```python
from build123d import *

# Parameters (mm, degrees)
SKETCH1_R             = 3.9
SKETCH1_R_2           = 1.5
BOSS_EXTRUDE1_DEPTH   = 10.061552014
BOSS_EXTRUDE1_2_DEPTH = 10.061552014
BOSS_EXTRUDE1_3_DEPTH = 10.061552014
BOSS_EXTRUDE1_4_DEPTH = 10.061552014
BOSS_EXTRUDE2_START   = 1.861552
SKETCH2_R             = 3.9
SKETCH2_R_2           = 9.3
BOSS_EXTRUDE2_DEPTH   = 10
CUT_EXTRUDE1_DEPTH    = 25
CUT_EXTRUDE2_DEPTH    = 72.170463178
SKETCH5_W             = 10
SKETCH5_H             = 10
SKETCH5_R             = 2
BOSS_EXTRUDE3_DEPTH   = 10


with BuildPart() as part:
    # Sketch1 → Boss-Extrude1 (new body)
    with BuildSketch(Plane.XY):
        with Locations(Location((-49, 7.83595021, 0), (0, 0, 180))):
            Circle(SKETCH1_R)
        with Locations(Location((-49, 7.83595021, 0), (0, 0, 180))):
            Circle(SKETCH1_R_2, mode=Mode.SUBTRACT)
    extrude(amount=BOSS_EXTRUDE1_DEPTH)



with BuildPart() as body_2:
    # Sketch1 → Boss-Extrude1 2 (new body)
    with BuildSketch(Plane.XY):
        with Locations(Location((-49, 35.83595021, 0), (0, 0, 180))):
            Circle(SKETCH1_R)
        with Locations(Location((-49, 35.83595021, 0), (0, 0, 180))):
            Circle(SKETCH1_R_2, mode=Mode.SUBTRACT)
    extrude(amount=BOSS_EXTRUDE1_2_DEPTH)


with BuildPart() as body_3:
    # Sketch1 → Boss-Extrude1 3 (new body)
    with BuildSketch(Plane.XY):
        with Locations(Location((-9, 35.83595021, 0), (0, 0, 180))):
            Circle(SKETCH1_R)
        with Locations(Location((-9, 35.83595021, 0), (0, 0, 180))):
            Circle(SKETCH1_R_2, mode=Mode.SUBTRACT)
    extrude(amount=BOSS_EXTRUDE1_3_DEPTH)


with BuildPart() as body_4:
    # Sketch1 → Boss-Extrude1 4 (new body)
    with BuildSketch(Plane.XY):
        with Locations(Location((-9, 7.83595021, 0), (0, 0, 180))):
            Circle(SKETCH1_R)
        with Locations(Location((-9, 7.83595021, 0), (0, 0, 180))):
            Circle(SKETCH1_R_2, mode=Mode.SUBTRACT)
    extrude(amount=BOSS_EXTRUDE1_4_DEPTH)


with BuildPart() as part_1:
    add(part.part)

    add(body_2.part)  # Boss-Extrude2 merges body 2

    add(body_3.part)  # Boss-Extrude2 merges body 3

    add(body_4.part)  # Boss-Extrude2 merges body 4
    # Sketch2 → Boss-Extrude2 (add)
    with BuildSketch(Plane.XY.offset(-1.8).offset(BOSS_EXTRUDE2_START)):
        Polygon((-58, 1.83595021), (0, 1.83595021), (0, 5.290014366), (0, 38.441339865), (0, 41.83595021), (-58, 41.83595021), align=None)
        with Locations(Location((-9, 35.83595021, 0), (0, 0, 180))):
            Circle(SKETCH2_R, mode=Mode.SUBTRACT)
        with Locations((-49, 7.83595021)):
            Circle(SKETCH2_R, mode=Mode.SUBTRACT)
        with Locations(Location((-38.5, 21.83595021, 0), (0, 0, 180))):
            Circle(SKETCH2_R_2, mode=Mode.SUBTRACT)
        with Locations(Location((-49, 35.83595021, 0), (0, 0, 180))):
            Circle(SKETCH2_R, mode=Mode.SUBTRACT)
        with Locations(Location((-9, 7.83595021, 0), (0, 0, 180))):
            Circle(SKETCH2_R, mode=Mode.SUBTRACT)
    extrude(amount=BOSS_EXTRUDE2_DEPTH)

    # Sketch4 → Cut-Extrude1 (cut)
    with BuildSketch(Plane(origin=(0, 41.83595021, 0), x_dir=(1, 0, 0), z_dir=(0, 1, 0))):
        with BuildLine():
            ThreePointArc((-23, -5.061552014), (-20, -8.061552014), (-17, -5.061552014))
            Line((-17, -5.061552014), (-18, -5.061552014))
            ThreePointArc((-18, -5.061552014), (-20, -7.061552014), (-22, -5.061552014))
            Line((-22, -5.061552014), (-23, -5.061552014))
        make_face()
        with BuildLine():
            Line((-18, -5.061552014), (-17, -5.061552014))
            ThreePointArc((-17, -5.061552014), (-20, -2.061552014), (-23, -5.061552014))
            Line((-23, -5.061552014), (-22, -5.061552014))
            ThreePointArc((-22, -5.061552014), (-20, -3.061552014), (-18, -5.061552014))
        make_face()
        with BuildLine():
            ThreePointArc((-22, -5.061552014), (-20, -7.061552014), (-18, -5.061552014))
            Line((-18, -5.061552014), (-22, -5.061552014))
        make_face()
        with BuildLine():
            Line((-22, -5.061552014), (-18, -5.061552014))
            ThreePointArc((-18, -5.061552014), (-20, -3.061552014), (-22, -5.061552014))
        make_face()
    extrude(amount=-CUT_EXTRUDE1_DEPTH, mode=Mode.SUBTRACT)

    # Sketch4<3> → Cut-Extrude2 (cut, through all)
    with BuildSketch(Plane(origin=(0, 41.83595021, 0), x_dir=(1, 0, 0), z_dir=(0, 1, 0))):
        with BuildLine():
            ThreePointArc((-22, -5.061552014), (-20, -7.061552014), (-18, -5.061552014))
            Line((-18, -5.061552014), (-22, -5.061552014))
        make_face()
        with BuildLine():
            Line((-22, -5.061552014), (-18, -5.061552014))
            ThreePointArc((-18, -5.061552014), (-20, -3.061552014), (-22, -5.061552014))
        make_face()
    extrude(amount=-CUT_EXTRUDE2_DEPTH, mode=Mode.SUBTRACT)

    # Sketch5 → Boss-Extrude3 (add)
    with BuildSketch(Plane(origin=(0, 1.83595021, 0), x_dir=(1, 0, 0), z_dir=(0, 1, 0))):
        with Locations((-63, -5.061552014)):
            Rectangle(SKETCH5_W, SKETCH5_H)
        with Locations(Location((-63, -5.061552014, 0), (0, 0, 180))):
            Circle(SKETCH5_R, mode=Mode.SUBTRACT)
    extrude(amount=BOSS_EXTRUDE3_DEPTH)


solid = part_1.part
```
For this review, take the finished solid that the model builds, in its own axes (mm). A direction names the side the tool comes from. Round coordinates to 2 decimals unless told otherwise and drop trailing zeros. Write each loop counter-clockwise with the first axis right and the second up, starting at its lowest first coordinate (ties: lowest second). Pieces come first, ordered by that corner, then holes. Notation, with made-up numbers: (-30, -40) -> (29, -40) arc R21 cw to (29, -12) -> close; hole circle Ø3 at (46, 60.5). An arc over 180 degrees is marked (long way). Use one line per item in the form item = value.
1) Take a section at C-C, the plane x = -41.5. Write out the cut boundary in (y, z).
Found:
outline = (1.84, 0.06) -> (13.03, 0.06) -> (13.03, 10.06) -> (1.84, 10.06) -> close; (30.64, 0.06) -> (41.84, 0.06) -> (41.84, 10.06) -> (30.64, 10.06) -> close
2) Take a section at A-A, the plane x = -9. Write out the cut boundary in (y, z).
Found:
outline = (1.84, 0.06) -> (3.94, 0.06) -> (3.94, 0) -> (6.34, 0) -> (6.34, 10.06) -> (1.84, 10.06) -> close; (9.34, 0) -> (11.74, 0) -> (11.74, 0.06) -> (31.94, 0.06) -> (31.94, 0) -> (34.34, 0) -> (34.34, 10.06) -> (9.34, 10.06) -> close; (37.34, 0) -> (39.74, 0) -> (39.74, 0.06) -> (41.84, 0.06) -> (41.84, 10.06) -> (37.34, 10.06) -> close
3) Mouldability with a two-part tool opening along X and no side actions: class faces 1 (the cylindrical face through (-47.5, 7.8, 5)), 2 (the flat face through (-34, 1.836, 5)), 3 (the flat face through (-58, 27, 5)) as +X half, -X half, draft (parallel to the pull), parting line (faces both ways), or undercut.
Found:
face_1 = undercut
face_2 = draft
face_3 = -X half
4) To check wall thickness, follow L1, parallel to Y at x = -9, z = 3.5; L2, parallel to Z at x = -20, y = 11; L3, parallel to Y at x = -38.5, z = 3.25. State the ranges of each line that lie inside material, in increasing order. Write a range as from..to.
Found:
L1 = 1.84..6.34, 9.34..34.34, 37.34..41.84
L2 = 0.06..3.06, 7.06..10.06
L3 = 1.84..12.54, 31.14..41.84
5) Tool access review of faces 4 (the flat face through (-27, 22, 10.062)), 5 (the flat face through (-18, 16.836, 6)), 6 (the flat face through (-65.3, 11.836, 5)), 7 (the cylindrical face through (-47.09, 25.4, 4.99)), 8 (the flat face through (-27, 22, 0.062)): name each direction out of +Z, -Z, +X, -X, +Y, -Y from which nothing blocks a thin tool from reaching the whole face with its end or side.
Found:
face_4 = +Z, +X, -X, +Y, -Y
face_5 = +Y
face_6 = +Z, -Z, -X, +Y
face_7 = +Z, -Z
face_8 = -Z
6) Clearance check with flat-ended pins moving along their axes: pin 1 (12 mm diameter, centred on x = -37.5, y = 28.5, fed in from -Z); pin 2 (4 mm diameter, centred on y = 15, z = 3, fed in from -X). State where each tip first meets the part, or that it passes through.
Found:
pin_1 = 0.06
pin_2 = -58
7) Take a section at B-B, the plane y = 29. Write out the cut boundary in (x, z).
Found:
outline = (-58, 0.06) -> (-44.43, 0.06) -> (-44.43, 10.06) -> (-58, 10.06) -> close; (-32.57, 0.06) -> (0, 0.06) -> (0, 10.06) -> (-32.57, 10.06) -> close; hole circle Ø6 at (-20, 5.06)
8) Take a section at D-D, the plane z = 9. Write out the cut boundary in (x, y), and give its area (3 significant figures).
Found:
outline = (-68, 1.84) -> (0, 1.84) -> (0, 41.84) -> (-58, 41.84) -> (-58, 11.84) -> (-68, 11.84) -> close; hole circle Ø3 at (-49, 7.84); hole circle Ø3 at (-49, 35.84); hole circle Ø18.6 at (-38.5, 21.84); hole circle Ø3 at (-9, 7.84); hole circle Ø3 at (-9, 35.84)
area = 2,120 mm2
